Source: CAD feature listing. Evaluate the final solid. Frame: model axes, mm. A direction names the side the tool comes from. Give positions to 0.01 mm unless a question says otherwise; leave off trailing zeros. Loops run counter-clockwise (first coordinate to the right, second up) from the corner with the lowest first, then second, coordinate; pieces in that order, holes last.
Autodesk Inventor part; units mm, degrees
ref_plane "YZ Plane" through (0, 0, 0) normal (1, 0, 0) x (0, 1, 0)
ref_plane "XZ Plane" through (0, 0, 0) normal (0, 1, 0) x (-1, 0, 0)
ref_plane "XY Plane" through (0, 0, 0) normal (0, 0, 1) x (1, 0, 0)
sketch "Sketch1" plane through (0, 0, 0) normal (0, 1, 0) x (-1, 0, 0)
  circle A0 centre (0, 0) radius 3
  dimension "d0" = 6
extrude "Extrusion1" add sketch "Sketch1" along normal blind 15
sketch "Sketch2" plane through (0, 15, 0) normal (0, 1, 0) x (1, 0, 0)
  point P0 (0, 0)
  point P1 (0, 0)
hole "Hole1" at (0, 15, 0) direction (0, -1, 0) diameter 2.156 depth 7.5 tip angle 118
sketch "Sketch3" plane through (0, 0, 0) normal (0, -1, 0) x (1, 0, 0)
  circle A0 centre (0, 0) radius 1.078
  circle A1 centre (0, 0) radius 0.85
  dimension "d10" = 1.7
extrude "Extrusion2" cut sketch "Sketch3" against normal blind 3.85 contours A1
sketch "Sketch4" plane through (0, 0, 0) normal (0, -1, 0) x (1, 0, 0)
  circle A0 centre (0, 0) radius 0.85
  circle A1 centre (0, 0) radius 3
  circle A2 centre (0, 0) radius 0.85
  circle A3 centre (0, 0) radius 0.875
  dimension "d13" = 1.75
extrude "Extrusion3" cut sketch "Sketch4" against normal blind 1.25 contours A3
properties part number "pin_adapter"
(1) Mould query, pull axis X, two halves, no side actions, for faces 1 (the cylindrical face through (3, 7, 0)), 2 (the flat face through (-1.3, 15, 0)), 3 (the cylindrical face through (0.808, 0.616, -0.335)). Classes: pulls with the +X half, pulls with the -X half, needs draft (parallel to the pull), parting line crosses it, or undercut.
A:
face 1: parting line crosses it
face 2: needs draft
face 3: undercut
(2) Reachability of faces 4 (the flat face through (0, 3.85, 0)), 5 (the flat face through (-1, 0, -1)), 6 (the cylindrical face through (-0.32, 11.2, 1.03)) from +Z, -Z, +X, -X, +Y, -Y: full face, straight path, thin tool, end or side. Return the list, or none.
A:
face 4: -Y
face 5: +Z, -Z, +X, -X, -Y
face 6: +Y
(3) First-contact query: pin 1 (2.5 mm diameter, centred on x = 0, z = 0, fed in from -Y); pin 2 (1 mm diameter, centred on y = 10.5, z = 1, fed in from -X); pin 3 (2 mm diameter, centred on x = 1.5, y = 9, fed in from -Z); pin 4 (1.4 mm diameter, centred on x = 0, z = 0, fed in from -Y). Flat tips, straight axial feed; report the tip coordinate or a pass-through.
A:
pin 1: stops at y = 0
pin 2: stops at x = -2.96
pin 3: stops at z = -2.96
pin 4: stops at y = 3.85
(4) Section C-C, the plane x = -1.7. Return the cut outline in (y, z).
A:
outline: (0, -2.47) - (15, -2.47) - (15, 2.47) - (0, 2.47) - close
(5) Section A-A, the plane y = 2. Return the cut outline in (x, z).
A:
outline: circle Ø6 at (0, 0); hole circle Ø1.7 at (0, 0)
(6) Ray query, line 1 along Z through (x, y) = (0, 11.5); line 2 along Z through (x, y) = (0, 2.3); line 3 along Z through (x, y) = (-0.1, 4). Return the intervals inside material, ascending.
A:
line 1: z = -3 to -1.08, 1.08 to 3
line 2: z = -3 to -0.85, 0.85 to 3
line 3: z = -3 to 3
(7) Section D-D, the plane z = -1.7. Return the cut outline in (x, y), then the cut area to 3 significant figures.
A:
outline: (-2.47, 0) - (2.47, 0) - (2.47, 15) - (-2.47, 15) - close
area: 74.2 mm2
(8) Section B-B, the plane y = 4.75. Return the cut outline in (x, z).
A:
outline: circle Ø6 at (0, 0)
